Work out the finished part from the listing and answer in its coordinate system (mm). Face numbers are marked on the shaded views. A direction names the side the tool comes from. Round coordinates to 2 decimals unless told otherwise and drop trailing zeros. Write each loop counter-clockwise with the first axis right and the second up, starting at its lowest first coordinate (ties: lowest second). Pieces come first, ordered by that corner, then holes. Notation, with made-up numbers: M 49,23 L 79,23 A22 ccw 79,47 Z; hole C 89.5,-14 d2. An arc over 180 degrees is marked long. One line per item, written item: value. Start each with the question number.
Q1. Find section A-A (x = 140). Write down the section's boundary in (y, z), and give its area (3 significant figures).
Q2. Find section C-C (z = -13). Write down the section's boundary in (x, y), and give its area (3 significant figures).
Q3. The mould has two halves that part along Y. Classify the marked faces 3, 4 and 5: released by +Y, released by -Y, zero draft, split by the parting line, or undercut.
Q4. Find section D-D (x = 14). Write down the section's boundary in (y, z), and give its area (3 significant figures).
Q5. Consider probe 1 along Y at (x, z) = (0, -9); probe 2 along X at (y, z) = (-3, -14); probe 3 along X at (y, z) = (1, -4.25). Determine where each line is inside the solid, lowest interval first.
Q6. Given pin 1 Ø2 at (y, z) = (-23, -13) entering from -X; pin 2 Ø1 at (x, z) = (121.5, -17) entering from -Y; pin 3 Ø4 at (x, z) = (-16.5, -16) entering from +Y, each flat-ended and moving along its own axis, determine where each tip first touches the part or whether it passes through.
Q7. Find section B-B (y = -2.5). Write down the section's boundary in (x, z).
Q8. A tool of negligible diameter and unlimited length cuts with its end or side. For the marked faces 1 and 2, from which of +Z, -Z, +X, -X, +Y, -Y can it reach the whole face along a straight path? Write none if from no direction.
from build123d import *

# Parameters (mm, degrees)
SKETCH1_R          = 30
SKETCH1_R_2        = 7
BASE_EXTRUDE_DEPTH = 20
FILLET1_R          = 10
FILLET2_R          = 20
CUT_EXTRUDE1_DEPTH = 5
CUT_EXTRUDE2_DEPTH = 21


with BuildPart() as part:
    # Sketch1 → Base-Extrude (new body)
    with BuildSketch(Plane.XY):
        with BuildLine():
            Line((27.935473676, 25.760615491), (128.063755469, 9.084385863))
            ThreePointArc((128.063755469, 9.084385863), (155, 0), (128.063755469, -9.084385863))
            Line((128.063755469, -9.084385863), (27.935473676, -25.760615491))
            ThreePointArc((27.935473676, -25.760615491), (-38, 0), (27.935473676, 25.760615491))
        make_face()
        Circle(SKETCH1_R, mode=Mode.SUBTRACT)
        with Locations((140, 0)):
            Circle(SKETCH1_R_2, mode=Mode.SUBTRACT)
    extrude(amount=-BASE_EXTRUDE_DEPTH)

    # Fillet1
    fillet1_edges = [part.edges().sort_by_distance(p)[0] for p in [
        (128.063755469, 9.084385863, -10),
        (128.063755469, -9.084385863, -10),
    ]]
    fillet(fillet1_edges, radius=FILLET1_R)

    # Fillet2
    fillet2_edges = [part.edges().sort_by_distance(p)[0] for p in [
        (27.935473676, 25.760615491, -10),
        (27.935473676, -25.760615491, -10),
    ]]
    fillet(fillet2_edges, radius=FILLET2_R)

    # Sketch2 → Cut-Extrude1 (cut)
    with BuildSketch(Plane.XY):
        with BuildLine():
            Line((41.828554558, 17.870982725), (121.046940728, 4.677267873))
            ThreePointArc((121.046940728, 4.677267873), (123.741079282, 3.147292859), (124.807655013, 0.238406077))
            ThreePointArc((124.807655013, 0.238406077), (123.914202634, -2.958553332), (121.071833732, -4.673121977))
            Line((121.071833732, -4.673121977), (41.828554558, -17.870982725))
            ThreePointArc((41.828554558, -17.870982725), (37.231968897, -16.217361812), (36.238855523, -11.43439331))
            ThreePointArc((36.238855523, -11.43439331), (38, 0), (36.238855523, 11.43439331))
            ThreePointArc((36.238855523, 11.43439331), (37.231968897, 16.217361812), (41.828554558, 17.870982725))
        make_face()
    extrude(amount=-CUT_EXTRUDE1_DEPTH, mode=Mode.SUBTRACT)

    # Sketch3 → Cut-Extrude2 (cut, through all)
    with BuildSketch(Plane(origin=(0, 0, -20), x_dir=(-1, 0, 0), z_dir=(0, 0, -1))):
        with BuildLine():
            Line((-121.445609231, 4.610870174), (-41.828554558, 17.870982725))
            ThreePointArc((-41.828554558, 17.870982725), (-37.231968897, 16.217361812), (-36.238855523, 11.43439331))
            ThreePointArc((-36.238855523, 11.43439331), (-38, 0), (-36.238855523, -11.43439331))
            ThreePointArc((-36.238855523, -11.43439331), (-37.231968897, -16.217361812), (-41.828554558, -17.870982725))
            Line((-41.828554558, -17.870982725), (-121.433526351, -4.612882562))
            ThreePointArc((-121.433526351, -4.612882562), (-124.132861899, -3.076762276), (-125.194211834, -0.157924451))
            ThreePointArc((-125.194211834, -0.157924451), (-124.244145959, 2.952985869), (-121.445609231, 4.610870174))
        make_face()
    extrude(amount=-CUT_EXTRUDE2_DEPTH, mode=Mode.SUBTRACT)


solid = part.part
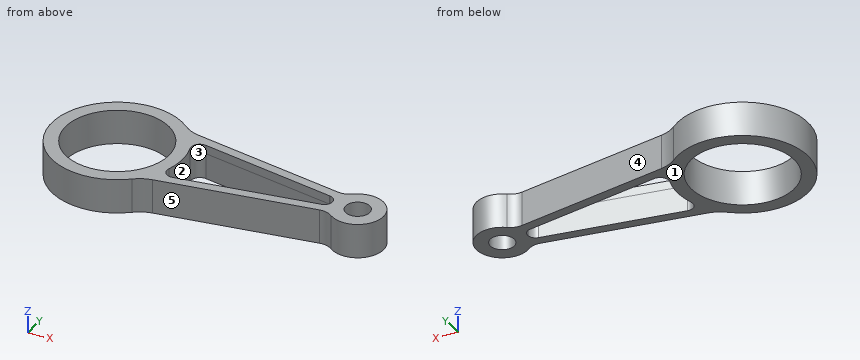
The answers:
1. outline: M -15,-20 L -7,-20 L -7,0 L -15,0 Z; M 7,-20 L 15,-20 L 15,0 L 7,0 Z
1. area: 320 mm2
2. outline: M 24.38,-29.15 A20 cw 33.92,-24.76 L 123.07,-9.92 A10 cw 130.83,-11.87 A15 ccw long 130.83,11.87 A10 cw 123.07,9.92 L 33.92,24.76 A20 cw 24.38,29.15 A38 ccw long Z; hole C 0,0 d60; hole M 36.24,-11.43 A5 ccw 41.83,-17.87 L 121.43,-4.61 A4.5 ccw 125.19,-0.16 A4.5 ccw 121.45,4.61 L 41.83,17.87 A5 ccw 36.24,11.43 A38 cw Z; hole C 140,0 d14
2. area: 3,390 mm2
3. face 3: undercut
3. face 4: released by +Y
3. face 5: released by -Y
4. outline: M -35.33,-20 L -26.53,-20 L -26.53,0 L -35.33,0 Z; M 26.53,-20 L 35.33,-20 L 35.33,0 L 26.53,0 Z
4. area: 352 mm2
5. probe 1: -38 to -30, 30 to 38
5. probe 2: -37.88 to -29.85, 29.85 to 37.88, 124.2 to 133.68, 146.32 to 154.7
5. probe 3: -37.99 to -29.98, 29.98 to 37.99, 125.13 to 133.07, 146.93 to 154.97
6. pin 1: x = -30.98
6. pin 2: y = -10.26
6. pin 3: y = 35.12
7. outline: M -37.92,-20 L -29.9,-20 L -29.9,0 L -37.92,0 Z; M 29.9,-20 L 37.92,-20 L 37.92,0 L 29.9,0 Z; M 124.55,-20 L 133.46,-20 L 133.46,0 L 124.55,0 Z; M 146.54,-20 L 154.79,-20 L 154.79,0 L 146.54,0 Z
8. face 1: -Z, +X, -X, +Y, -Y
8. face 2: +Z, -Z
